Part model, mm, in its own coordinate system. Face numbers are marked on the shaded views. Coordinates: 2 decimals unless noted, no trailing zeros. Loops run counter-clockwise (first coordinate to the right, second up) from the corner with the lowest first, then second, coordinate; pieces in that order, holes last. Notation, with made-up numbers: (81.5, 88.25) -> (91.5, 88.25) arc R36 cw to (91.5, 126.25) -> close; hole circle Ø4 at (53, 76). An arc over 180 degrees is marked (long way). One line per question, with ' | ' between items. Start each with the question number.
1) Two-plate mould, pull along Y, no slides. Class the marked faces 1 and 2: released by +Y, released by -Y, zero draft, split by the parting line, or undercut.
2) Cut at B-B (x = -19). List the corners of the cut face in (y, z), plus the area to 3 significant figures.
3) Drop flat-ended pins along their axis: pin 1 (1.5 mm diameter, centred on y = 32.5, z = 17, fed in from -X); pin 2 (2.5 mm diameter, centred on x = -19, z = 16.5, fed in from +Y); pin 3 (3 mm diameter, centred on x = 6, z = 18.5, fed in from -Y) (3 decimals). Give the stop position or say it passes through.
4) Probe L1, parallel to X at y = 7, z = 16.25; L2, parallel to X at y = 52, z = 18.05; L3, parallel to Y at x = 16.5, z = 18.95. List the from-to ranges inside material, lowest first. Write a range as from..to.
5) Cut at A-A (z = 15.6). List the corners of the cut face in (x, y).
from build123d import *

# Parameters (mm, degrees)
F1_ANGLE = 90
F3_DEPTH = 25
F5_DEPTH = 3


with BuildPart() as f1:
    # F0 (on Front) → F1 (revolve)
    with BuildSketch(Plane.XZ):
        Polygon((52.5206645727, 17.0954047681), (52.5206645727, 14.0954047681), (82.5206645727, 14.0954047681), (82.5206645727, 17.0954047681), (81.5206645727, 17.0954047681), (77.5206645727, 17.0954047681), (57.5206645727, 17.0954047681), (53.5206645727, 17.0954047681), align=None)
        Polygon((77.5206645727, 17.0954047681), (81.5206645727, 17.0954047681), (81.5206645727, 17.5954047681), (80.5206645727, 19.5954047681), (78.5206645727, 19.5954047681), (77.5206645727, 17.5954047681), align=None)
        Polygon((53.5206645727, 17.5954047681), (53.5206645727, 17.0954047681), (57.5206645727, 17.0954047681), (57.5206645727, 17.5954047681), (56.5206645727, 19.5954047681), (54.5206645727, 19.5954047681), align=None)
    revolve(axis=Axis((-17.4793354273, 0, 16.5954047681), (0, 0, 1)), revolution_arc=F1_ANGLE)

    # F2 (on face) → F3 (cut)
    with BuildSketch(Plane(origin=(0, 0, 14.0954047681), x_dir=(1, 0, 0), z_dir=(0, 0, -1))):
        with BuildLine():
            ThreePointArc((70.7706645727, -3.2003289616), (69.2529527716, -2.3096719096), (67.5206645727, -2))
            ThreePointArc((67.5206645727, -2), (65.7883763738, -2.3096719096), (64.2706645727, -3.2003289616))
            ThreePointArc((64.2706645727, -3.2003289616), (65.4290145064, -11.5414755311), (72.5206645727, -7))
            ThreePointArc((72.5206645727, -7), (72.0621401039, -4.9083499337), (70.7706645727, -3.2003289616))
        make_face()
        with BuildLine():
            Line((67.5206645727, -2), (67.5206645727, 0))
            Line((67.5206645727, 0), (64.2706645727, 0))
            Line((64.2706645727, 0), (64.2706645727, -3.2003289616))
            ThreePointArc((64.2706645727, -3.2003289616), (65.7883763738, -2.3096719096), (67.5206645727, -2))
        make_face()
        with BuildLine():
            Line((70.7706645727, 0), (67.5206645727, 0))
            Line((67.5206645727, 0), (67.5206645727, -2))
            ThreePointArc((67.5206645727, -2), (69.2529527716, -2.3096719096), (70.7706645727, -3.2003289616))
            Line((70.7706645727, -3.2003289616), (70.7706645727, 0))
        make_face()
    extrude(amount=-F3_DEPTH, mode=Mode.SUBTRACT)

    # F4 (on face) → F5 (join)
    with BuildSketch(Plane(origin=(0, 0, 14.0954047681), x_dir=(1, 0, 0), z_dir=(0, 0, -1))):
        with BuildLine():
            Line((-17.4793354273, -88), (-17.4793354273, -85))
            Line((-17.4793354273, -85), (-19.7293354273, -85))
            ThreePointArc((-19.7293354273, -85), (-20.0040998281, -86.5920949505), (-20.7966054616, -88))
            Line((-20.7966054616, -88), (-17.4793354273, -88))
        make_face()
        with BuildLine():
            Line((-19.7293354273, -85), (-17.4793354273, -85))
            Line((-17.4793354273, -85), (-17.4793354273, -82))
            Line((-17.4793354273, -82), (-20.7966054616, -82))
            ThreePointArc((-20.7966054616, -82), (-20.0040998281, -83.4079050495), (-19.7293354273, -85))
        make_face()
        with BuildLine():
            ThreePointArc((-20.7966054616, -88), (-20.0040998281, -86.5920949505), (-19.7293354273, -85))
            ThreePointArc((-19.7293354273, -85), (-20.0040998281, -83.4079050495), (-20.7966054616, -82))
            ThreePointArc((-20.7966054616, -82), (-29.2293354273, -85), (-20.7966054616, -88))
        make_face()
    extrude(amount=-F5_DEPTH)


solid = f1.part
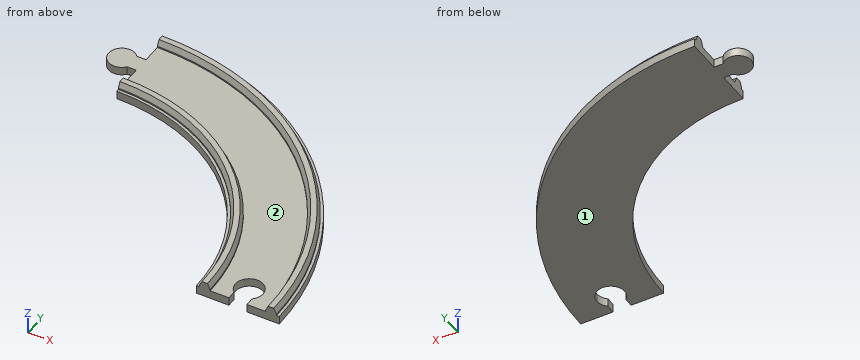
Reported:
1) face 1: zero draft | face 2: undercut
2) outline: (82, 14.1) -> (88, 14.1) -> (88, 17.1) -> (82, 17.1) -> close | area: 18.0 mm²
3) pin 1: stops at x = 44.12 | pin 2: stops at y = 88 | pin 3: stops at y = 65.755
4) L1: x = 52.17..62.52, 72.52..82.28 | L2: x = 31.2..36.25, 62.3..66.5 | L3: y = 63.11..66.1, 89.44..92.26
5) outline: (-20.8, 82) -> (-17.48, 82) -> (-17.48, 70) arc R70 cw to (52.52, 0) -> (64.27, 0) -> (64.27, 3.2) arc R5 cw (long way) to (70.77, 3.2) -> (70.77, 0) -> (82.52, 0) arc R100 ccw to (-17.48, 100) -> (-17.48, 88) -> (-20.8, 88) arc R4.75 ccw (long way) to start
